Answer from the drawing. Dimensions are ordinates in mm from the lowest x, y and z of the part. A direction names the side the tool comes from. Round coordinates to 2 decimals unless told otherwise and drop trailing zeros. Loops run counter-clockwise (first coordinate to the right, second up) from the corner with the lowest first, then second, coordinate; pieces in that order, holes last. Notation, with made-up numbers: M 27.25,-17.75 L 44.25,-17.75 A24 ccw 44.25,14.25 Z; hole C -19.5,-10.75 d10. An arc over 180 degrees is marked long. Answer as CSV lines item,"result".
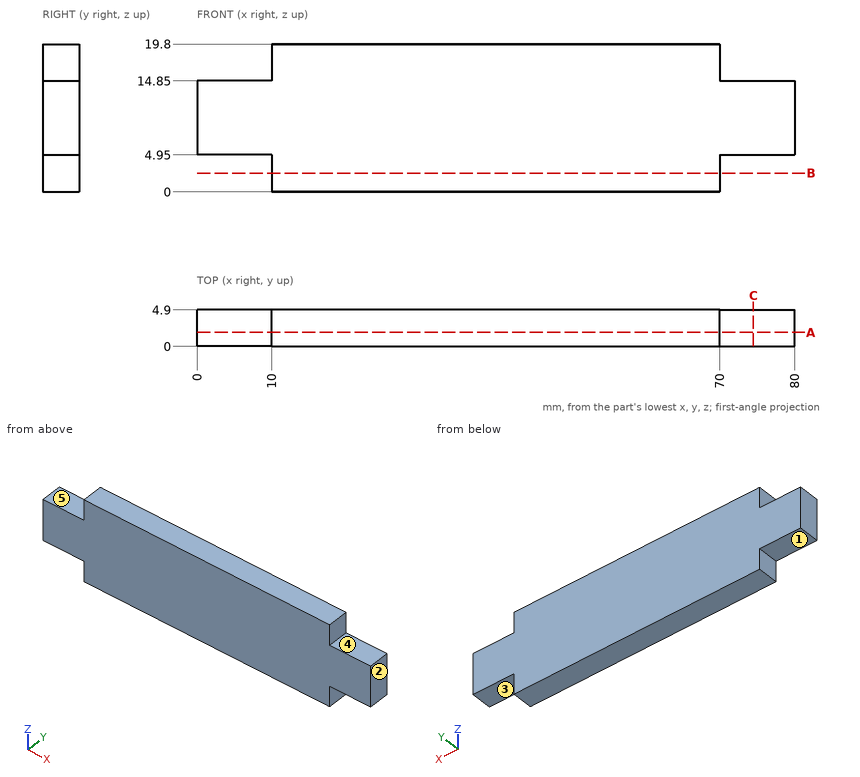
1) Find section A-A, the plane y = 1.9. Give the vertices of the cut face in (x, z), then the cut area to 3 significant figures.
Evaluation:
outline,"M 0,4.95 L 10,4.95 L 10,0 L 70,0 L 70,4.95 L 80,4.95 L 80,14.85 L 70,14.85 L 70,19.8 L 10,19.8 L 10,14.85 L 0,14.85 Z"
area,"1,390 mm^2"
2) A tool of negligible diameter and unlimited length cuts with its end or side. For the marked faces 1, 2, 3, 4 and 5, from which of +Z, -Z, +X, -X, +Y, -Y can it reach the whole face along a straight path? Write none if from no direction.
Evaluation:
face 1,"-Z, -X, +Y, -Y"
face 2,"+Z, -Z, +X, +Y, -Y"
face 3,"-Z, +X, +Y, -Y"
face 4,"+Z, +X, +Y, -Y"
face 5,"+Z, -X, +Y, -Y"
3) Each of these flat-tipped pins is pushed along its axis until it touches: P1, Ø1.5, axis at x = 7, y = 3, coming from the +Z side; P2, Ø2.5, axis at y = 1.5, z = 16.5, coming from the +X side; P3, Ø1.5, axis at y = 2, z = 5.5, coming from the -X side. Where does it stop, or does it pass through?
Evaluation:
P1,"stops at z = 14.85"
P2,"stops at x = 70"
P3,"stops at x = 0"
4) Find section C-C, the plane x = 74.5. Give the vertices of the cut face in (y, z), then the cut area to 3 significant figures.
Evaluation:
outline,"M 0,4.95 L 4.9,4.95 L 4.9,14.85 L 0,14.85 Z"
area,"48.5 mm^2"
5) Straight lines are drawn through the part: line 1 (X direction, y = 4.55, z = 4); line 2 (Z direction, x = 72, y = 4.3). For each, find the intervals that lie inside material, in ascending order.
Evaluation:
line 1,"x = 10 to 70"
line 2,"z = 4.95 to 14.85"
6) Find section B-B, the plane z = 2.5. Give the vertices of the cut face in (x, y), then the cut area to 3 significant figures.
Evaluation:
outline,"M 10,0 L 70,0 L 70,4.9 L 10,4.9 Z"
area,"294 mm^2"
